```python
from build123d import *

# Parameters (mm, degrees)
SALIENTE_EXTRUIR1_DEPTH = 14
CROQUIS3_R              = 11.25
CORTAR_EXTRUIR1_DEPTH   = 7
CROQUIS4_R              = 9
CORTAR_EXTRUIR2_DEPTH   = 1
CORTAR_EXTRUIR3_REACH   = 112.059
CROQUIS5_R              = 6
CROQUIS8_W              = 10
CROQUIS8_H              = 32
SALIENTE_EXTRUIR4_DEPTH = 20
REDONDEO1_R             = 5
CROQUIS10_W             = 60
CROQUIS10_H             = 6
SALIENTE_EXTRUIR7_DEPTH = 1
CROQUIS6_R              = 2.75
CORTAR_EXTRUIR6_DEPTH   = 40
CROQUIS11_R             = 6
CORTAR_EXTRUIR7_DEPTH   = 8


with BuildPart() as part:
    # Croquis2 → Saliente-Extruir1 (new body)
    with BuildSketch(Plane.XY):
        Polygon((0, 0), (-105, 0), (-105, -32), (-60, -32), (-60, -20), (0, -20), align=None)
    extrude(amount=SALIENTE_EXTRUIR1_DEPTH)

    # Croquis3 → Cortar-Extruir1 (cut)
    with BuildSketch(Plane.XY.offset(14)):
        with Locations((-89, -16)):
            Circle(CROQUIS3_R)
    extrude(amount=-CORTAR_EXTRUIR1_DEPTH, mode=Mode.SUBTRACT)

    # Croquis4 → Cortar-Extruir2 (cut)
    with BuildSketch(Plane.XY.offset(7)):
        with Locations((-89, -16)):
            Circle(CROQUIS4_R)
    extrude(amount=-CORTAR_EXTRUIR2_DEPTH, mode=Mode.SUBTRACT)

    # Croquis5 → Cortar-Extruir3 (cut, up to next)
    with BuildSketch(Plane.XY.offset(6), mode=Mode.PRIVATE) as cortar_extruir3_sk1:
        with Locations((-89, -16)):
            Circle(CROQUIS5_R)
    cortar_extruir3_tool1 = extrude(cortar_extruir3_sk1.sketch, amount=-CORTAR_EXTRUIR3_REACH, mode=Mode.PRIVATE) & part.part
    add(cortar_extruir3_tool1.solids().sort_by_distance((-89, -16, 6))[0], mode=Mode.SUBTRACT)

    # Croquis8 → Saliente-Extruir4 (add)
    with BuildSketch(Plane.XY.offset(14)):
        with Locations((-65, -16)):
            Rectangle(CROQUIS8_W, CROQUIS8_H)
    extrude(amount=SALIENTE_EXTRUIR4_DEPTH)

    # Redondeo1
    redondeo1_edges = [part.edges().sort_by_distance(p)[0] for p in [
        (-70, 0, 24),
        (-70, -32, 24),
        (-60, -20, 7),
        (-105, -32, 7),
        (-105, 0, 7),
        (-60, -32, 17),
    ]]
    fillet(redondeo1_edges, radius=REDONDEO1_R - 0.0001)  # a hair under: the kernel refuses the full size

    # Croquis10 → Saliente-Extruir7 (add)
    with BuildSketch(Plane.XY.offset(14)):
        with Locations((-30, -10)):
            Rectangle(CROQUIS10_W, CROQUIS10_H)
    extrude(amount=SALIENTE_EXTRUIR7_DEPTH)

    # Croquis6 → Cortar-Extruir6 (cut)
    with BuildSketch(Plane(origin=(0, 0, 0), x_dir=(-1, 0, 0), z_dir=(0, 0, -1))):
        with Locations((10, -10)):
            Circle(CROQUIS6_R)
        with Locations((30, -10)):
            Circle(CROQUIS6_R)
        with Locations((50, -10)):
            Circle(CROQUIS6_R)
    extrude(amount=-CORTAR_EXTRUIR6_DEPTH, mode=Mode.SUBTRACT)

    # Croquis11 → Cortar-Extruir7 (cut)
    with BuildSketch(Plane(origin=(0, 0, 0), x_dir=(-1, 0, 0), z_dir=(0, 0, -1))):
        with Locations((10, -10)):
            Circle(CROQUIS11_R)
        with Locations((30, -10)):
            Circle(CROQUIS11_R)
        with Locations((50, -10)):
            Circle(CROQUIS11_R)
    extrude(amount=-CORTAR_EXTRUIR7_DEPTH, mode=Mode.SUBTRACT)


solid = part.part
```
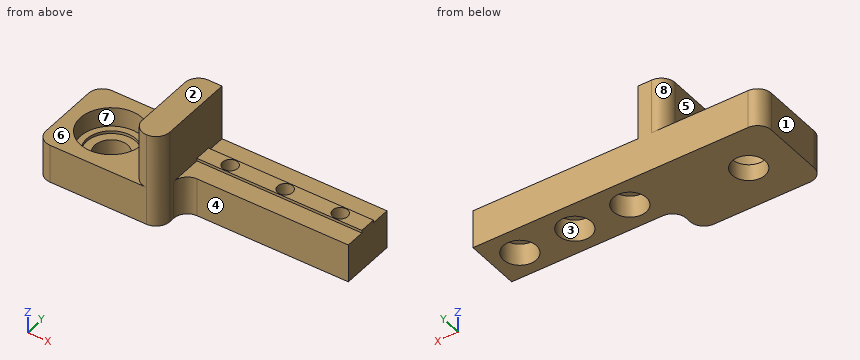
Source: CAD feature listing. Evaluate the final solid. Frame: model axes, mm. Face numbers are marked on the shaded views. A direction names the side the tool comes from. Round coordinates to 2 decimals unless told otherwise and drop trailing zeros. Write each loop counter-clockwise with the first axis right and the second up, starting at its lowest first coordinate (ties: lowest second). Pieces come first, ordered by that corner, then holes. Notation, with made-up numbers: M 52,-35 L 73,-35 A25 ccw 73,4 Z; hole C 40.25,7.25 d10. An arc over 180 degrees is marked long. Answer as a JSON object with one key per item and string values. Group by question number.
(1) Section query A-A on x = -10. Output: boundary loops of the cut face in (y, z).
(2) Section query D-D on x = -22. Output: boundary loops of the cut face in (y, z), then the cut area to 3 significant figures.
(3) Ray query, line 1 (Y direction, x = -30, z = 4); line 2 (Y direction, x = -10, z = 12); line 3 (Z direction, x = -19, y = -14.5). Return the intervals inside material, ascending. Write a range as [from, to].
(4) First-contact query: pin 1 (6.5 mm diameter, centred on x = -36.5, y = -10, fed in from +Z); pin 2 (9.5 mm diameter, centred on x = -10.5, y = -11, fed in from -Z); pin 3 (16 mm diameter, centred on x = -89, y = -16, fed in from +Z). Flat tips, straight axial feed; report the tip coordinate or a pass-through.
(5) Mould query, pull axis X, two halves, no side actions, for the marked faces 6, 7 and 8. Classes: +X half, -X half, draft (parallel to the pull), parting line (faces both ways), or undercut.
(6) Reachability of the marked faces 1, 2, 3, 4 and 5 from +Z, -Z, +X, -X, +Y, -Y: full face, straight path, thin tool, end or side. Return the list, or none.
(7) Section query B-B on z = 10.5. Output: boundary loops of the cut face in (x, y), then the cut area to 3 significant figures.
Computed values:
{
 "1": {"outline": "M -20,0 L -16,0 L -16,8 L -12.75,8 L -12.75,15 L -13,15 L -13,14 L -20,14 Z; M -7.25,8 L -4,8 L -4,0 L 0,0 L 0,14 L -7,14 L -7,15 L -7.25,15 Z"},
 "2": {"outline": "M -20,0 L 0,0 L 0,14 L -7,14 L -7,15 L -13,15 L -13,14 L -20,14 Z", "area": "286 mm^2"},
 "3": {"line 1": "[-20, -16], [-4, 0]", "line 2": "[-20, -12.75], [-7.25, 0]", "line 3": "[0, 14]"},
 "4": {"pin 1": "z = 15", "pin 2": "z = 8", "pin 3": "z = 6"},
 "5": {"face 6": "draft", "face 7": "undercut", "face 8": "-X half"},
 "6": {"face 1": "+Z, -Z, -X, +Y, -Y", "face 2": "+Z, +X, -X, +Y, -Y", "face 3": "-Z", "face 4": "+Z, -Z, +X, -Y", "face 5": "+Z, -X, +Y, -Y"},
 "7": {"outline": "M -105,-27 A5 ccw -100,-32 L -65,-32 A5 ccw -60,-27 L -60,-25 A5 cw -55,-20 L 0,-20 L 0,0 L -100,0 A5 ccw -105,-5 Z; hole C -89,-16 d22.5; hole C -50,-10 d5.5; hole C -30,-10 d5.5; hole C -10,-10 d5.5", "area": "2,160 mm^2"}
}
